Verification items for this drawing (mm, ordinates from the low corner). Coordinates: 2 decimals unless noted, no trailing zeros. Order: outer loops, then holes, each group sorted by start corner. A loop starts at its lowest first (then second) coordinate and runs counter-clockwise, first axis right, second up. Notation, with made-up numbers: (76.5, -30) -> (94.5, -30) arc R25 cw to (94.5, -14) -> close; hole circle Ø5 at (-7, 57). An arc over 180 degrees is marked (long way). Write each question's results on one line, items separated by ' | '. Start each with the question number.
(1) Thickness scan on probe 1 along Y at (x, z) = (33, 7.75) (1 decimal); probe 2 along Y at (x, z) = (38.5, 15.25); probe 3 along Z at (x, y) = (39, 159.5). Record the ranges inside material, lowest first. Write a range as [from, to].
(2) Cross-section at A-A on y = 89.5. Enter the section's corners in (x, z).
(3) Cross-section at B-B on x = 70.5. Enter the section's corners in (y, z), and give its area (3 significant figures).
(4) Go/stop test with a flat-tipped pin: pin 1 (8.5 mm diameter, centred on x = 38.6, y = 7.32, fed in from -Z). Record where the tip stops, or that it passes through.
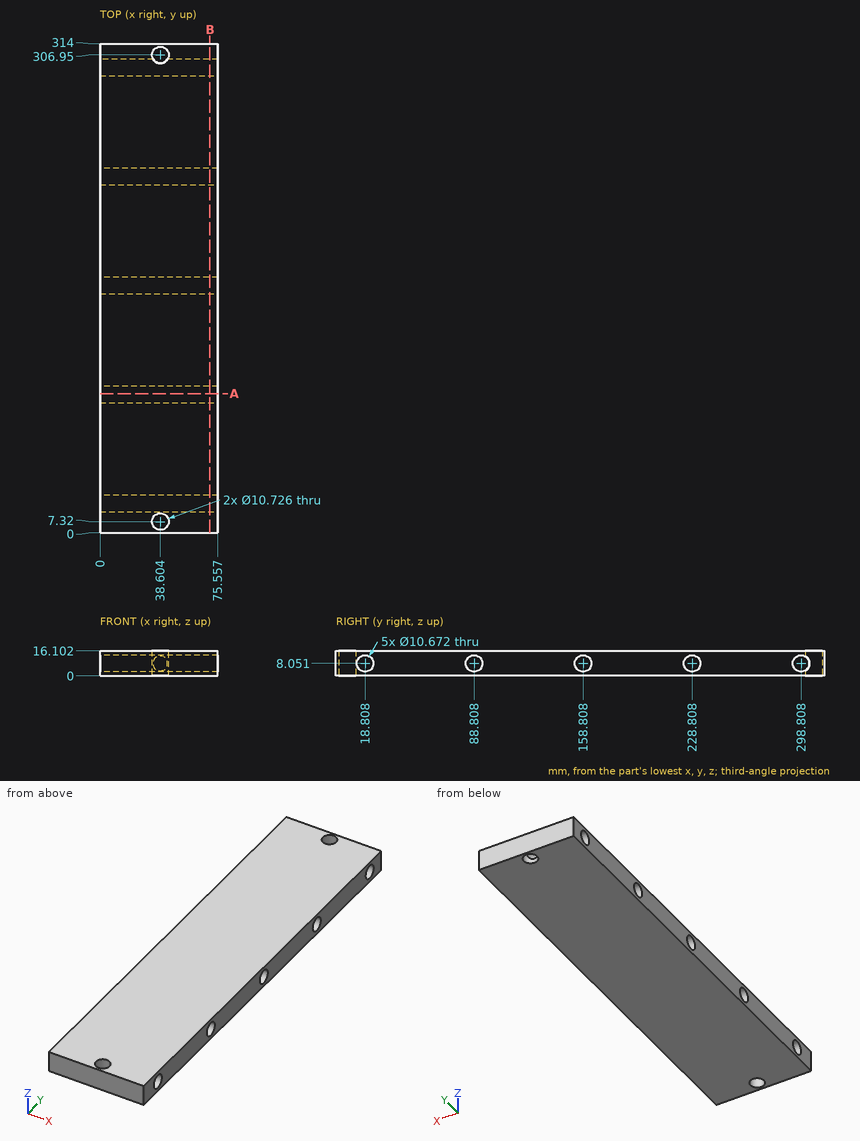
Results are:
1) probe 1: y = [0, 13.5], [24.1, 83.5], [94.1, 153.5], [164.1, 223.5], [234.1, 293.5], [304.1, 314] | probe 2: y = [0, 1.96], [12.68, 301.59], [312.31, 314] | probe 3: z = [0, 2.76], [13.34, 16.1]
2) outline: (0, 0) -> (75.56, 0) -> (75.56, 2.76) -> (0, 2.76) -> close; (0, 13.34) -> (75.56, 13.34) -> (75.56, 16.1) -> (0, 16.1) -> close
3) outline: (0, 0) -> (314, 0) -> (314, 16.1) -> (0, 16.1) -> close; hole circle Ø10.67 at (18.81, 8.05); hole circle Ø10.67 at (88.81, 8.05); hole circle Ø10.67 at (158.81, 8.05); hole circle Ø10.67 at (228.81, 8.05); hole circle Ø10.67 at (298.81, 8.05) | area: 4,610 mm2
4) pin 1: passes through
